Autodesk Fusion 360 part; units mm, degrees
sketch "Szkic1" plane through (0, 0, 0) normal (0, 0, 1) x (1, 0, 0)
  line L0 (0, 0) -> (75, 0)
  line L1 (75, 0) -> (75, 12)
  line L2 (75, 12) -> (0, 12)
  line L3 (0, 12) -> (0, 0)
  dimension "d1" = 75
  dimension "d2" = 12
extrude "Wyciągnięcie proste1" add sketch "Szkic1" along normal blind 2
sketch "Szkic2" plane through (0, 0, 2) normal (0, 0, 1) x (-1, 0, 0)
  line L0 (0, -12) -> (0, 0)
  line L1 (0, 0) -> (-75, 0)
  line L2 (-75, 0) -> (-75, -12)
  line L3 (-75, -12) -> (0, -12)
  line L4 (-3, -1) -> (-5, -1)
  line L5 (-5, -1) -> (-5, -4)
  line L6 (-5, -4) -> (-3, -4)
  line L7 (-3, -4) -> (-3, -1)
  line L8 (-72, -1) -> (-70, -1)
  line L9 (-70, -1) -> (-70, -4)
  line L10 (-70, -4) -> (-72, -4)
  line L11 (-72, -4) -> (-72, -1)
  line L12 (-12, -1) -> (-14, -1)
  line L13 (-14, -1) -> (-14, -4)
  line L14 (-14, -4) -> (-12, -4)
  line L15 (-12, -4) -> (-12, -1)
  line L16 (-63, -1) -> (-61, -1)
  line L17 (-61, -1) -> (-61, -4)
  line L18 (-61, -4) -> (-63, -4)
  line L19 (-63, -4) -> (-63, -1)
  line L20 (-22, -1) -> (-24, -1)
  line L21 (-24, -1) -> (-24, -4)
  line L22 (-24, -4) -> (-22, -4)
  line L23 (-22, -4) -> (-22, -1)
  line L24 (-53, -1) -> (-51, -1)
  line L25 (-51, -1) -> (-51, -4)
  line L26 (-51, -4) -> (-53, -4)
  line L27 (-53, -4) -> (-53, -1)
  line L28 (-32, -1) -> (-34, -1)
  line L29 (-34, -1) -> (-34, -4)
  line L30 (-34, -4) -> (-32, -4)
  line L31 (-32, -4) -> (-32, -1)
  line L32 (-43, -1) -> (-41, -1)
  line L33 (-41, -1) -> (-41, -4)
  line L34 (-41, -4) -> (-43, -4)
  line L35 (-43, -4) -> (-43, -1)
extrude "Wyciągnięcie proste2" add sketch "Szkic2" along normal blind 2 contours L4 L5 L6 L7 | L8 L9 L10 L11 | L12 L13 L14 L15 | L16 L17 L18 L19 | L20 L21 L22 L23 | L24 L25 L26 L27 | L28 L29 L30 L31 | L32 L33 L34 L35
sketch "Szkic3" plane through (0, 0, 0) normal (0, 0, -1) x (1, 0, 0)
  line L0 (0, 0) -> (0, -12)
  line L1 (0, -12) -> (75, -12)
  line L2 (75, -12) -> (75, 0)
  line L3 (75, 0) -> (0, 0)
  circle A0 centre (2.5, -10) radius 1
  circle A1 centre (72.5, -10) radius 1
  dimension "d8" = 2
  dimension "d9" = 2
extrude "Wyciągnięcie proste3" cut sketch "Szkic3" against normal blind 4 contours A0 | A1
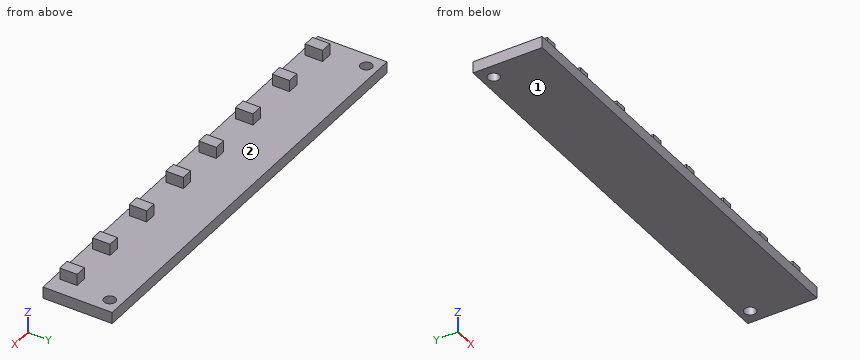
Can you work these out from the model? Positions are in its coordinate system, mm. Face numbers are marked on the shaded views. Coordinates: 2 decimals unless noted, no trailing zeros. Write each loop counter-clockwise with the first axis right and the second up, starting at its lowest first coordinate (ties: lowest second). Pieces come first, ordered by that corner, then holes. Notation, with made-up numbers: (-3.5, 36.5) -> (30.5, 36.5) arc R30 cw to (30.5, 61.5) -> close; hole circle Ø7 at (86.25, -34.5). An arc over 180 degrees is marked (long way). Write item = value, one per line.
(1) For pin 1 (1 mm diameter, centred on y = 2.5, z = 3, fed in from +X); pin 2 (2 mm diameter, centred on y = 2, z = 3.5, fed in from -X); pin 3 (1.6 mm diameter, centred on x = 71.5, z = 3.5, fed in from +Y), each with a flat end and sliding along its axis, tell me the tip position at first contact or that it passes through.
Verdict:
pin_1 = 72
pin_2 = 3
pin_3 = 4
(2) If I drill on probe 1 along X at (y, z) = (10, 0.5); probe 2 along Y at (x, z) = (2.5, 0.85); probe 3 along Z at (x, y) = (38, 10.75), over which ranges is the centre line in solid material (lowest first)?
Verdict:
probe_1 = 0 to 1.5, 3.5 to 71.5, 73.5 to 75
probe_2 = 0 to 9, 11 to 12
probe_3 = 0 to 2
(3) Imagine slicing it at B-B (x = 59). Please give me the cut outline in (y, z), and give its area (3 significant figures).
Verdict:
outline = (0, 0) -> (12, 0) -> (12, 2) -> (0, 2) -> close
area = 24.0 mm^2
(4) Thinking about a two-plate mould opening in X: for the marked faces 1 and 2, which applies, +X half, -X half, draft (parallel to the pull), parting line (faces both ways), or undercut?
Verdict:
face_1 = draft
face_2 = undercut
(5) Imagine slicing it at A-A (y = 10). Please give me the cut outline in (x, z), and give its area (3 significant figures).
Verdict:
outline = (0, 0) -> (1.5, 0) -> (1.5, 2) -> (0, 2) -> close; (3.5, 0) -> (71.5, 0) -> (71.5, 2) -> (3.5, 2) -> close; (73.5, 0) -> (75, 0) -> (75, 2) -> (73.5, 2) -> close
area = 142 mm^2
